Here's how the part is built. I have some questions about the finished solid (model axes, mm). A direction names the side the tool comes from. Coordinates: 2 decimals unless noted, no trailing zeros. Write each loop counter-clockwise with the first axis right and the second up, starting at its lowest first coordinate (ties: lowest second). Pieces come first, ordered by that corner, then holes.
Item 1: I want a section at C-C (y = -3). Please give me the cut outline in (x, z), and give its area (3 significant figures).
Item 2: I'm going to push flat-ended pins straight in: P1, Ø1.5, axis at x = 5, z = -1.5, coming from the -Y side; P2, Ø3, axis at y = -4, z = -2, coming from the -X side; P3, Ø1.5, axis at y = -18, z = 2.5, coming from the -X side; P4, Ø1, axis at y = 2, z = 1.5, coming from the -X side. Where does each tip first touch, or does it pass through?
Item 3: If we mould it in two halves opening along Y, with no side actions, what happens to faces 5 (the face through (-15, -7, 2)), 6 (the face through (-13.5, 5.07, 2.54)), 7 (the face through (10, -2, 1))? For each: pulls with the +Y half, pulls with the -Y half, needs draft (parallel to the pull), parting line crosses it, or undercut.
Item 4: I want a section at B-B (x = 18.5). Please give me the cut outline in (y, z), and give its area (3 significant figures).
Item 5: Please list where these lines run through material, in increasing order: line 1 (X direction, y = -13.5, z = 2.5); line 2 (X direction, y = -6.25, z = 1); line 3 (X direction, y = -7.75, z = 2).
Item 6: For faces 1 (the face through (8.4, -3.7, 3)), 2 (the face through (15.5, -3, -2)), 3 (the face through (-1, -14.5, 2)), 4 (the face through (8.84, -5.94, -1.97)), which set-ups out of +Z, -Z, +X, -X, +Y, -Y let a thin tool reach every point of the face, with its end or its side?
Item 7: I want a section at D-D (x = -7.5). Please give me the cut outline in (y, z), and give its area (3 significant figures).
from build123d import *

# Parameters (mm, degrees)
SKETCH1_W             = 23
SKETCH1_H             = 21
EXTRUDE1_DEPTH        = 5
SKETCH2_R             = 2.15
EXTRUDE2_DEPTH        = 4.3
SKETCH3_R             = 4.5
EXTRUDE3_DEPTH        = 4.5
SKETCH4_R             = 1.25
EXTRUDE4_DEPTH        = 8
SKETCH7_W             = 12
SKETCH7_H             = 26
EXTRUDE6_DEPTH        = 5
SKETCH9_R             = 1.5
EXTRUDE8_DEPTH        = 5
SKETCH8_R             = 2
EXTRUDE7_DEPTH        = 4
FILLET2_R             = 3
M3_TAPPED_HOLE1_D     = 2.5
M3_TAPPED_HOLE1_DEPTH = 8
M3_TAPPED_HOLE1_TIP   = 0.751075774
EXTRUDE9_DEPTH        = 4
FILLET1_R             = 5
EXTRUDE10_DEPTH       = 4
FILLET3_R             = 2


with BuildPart() as part:
    # Sketch1 → Extrude1 (new body)
    with BuildSketch(Plane.XY):
        with Locations((-3.5, -4)):
            Rectangle(SKETCH1_W, SKETCH1_H)
    extrude(amount=EXTRUDE1_DEPTH)

    # Sketch2 → Extrude2 (cut)
    with BuildSketch(Plane.XY.offset(5)):
        with Locations((-6, 0)):
            Circle(SKETCH2_R)
    extrude(amount=-EXTRUDE2_DEPTH, mode=Mode.SUBTRACT)

    # Sketch3 → Extrude3 (cut)
    with BuildSketch(Plane(origin=(0, 0, 0), x_dir=(-1, 0, 0), z_dir=(0, 0, -1))):
        with Locations((4.9, -6.5)):
            Circle(SKETCH3_R)
    extrude(amount=-EXTRUDE3_DEPTH, mode=Mode.SUBTRACT)

    # Sketch4 → Extrude4 (cut)
    with BuildSketch(Plane.XZ.offset(14.5)):
        with Locations(Location((-12, 2.5, 0), (0, 0, 270))):
            Circle(SKETCH4_R)
        with Locations(Location((1.4, 2.5, 0), (0, 0, 270))):
            Circle(SKETCH4_R)
    extrude(amount=-EXTRUDE4_DEPTH, mode=Mode.SUBTRACT)

    # Sketch7 → Extrude6 (add)
    with BuildSketch(Plane.XY.offset(5)):
        with Locations((14, -6.5)):
            Rectangle(SKETCH7_W, SKETCH7_H)
    extrude(amount=-EXTRUDE6_DEPTH)

    # Sketch9 → Extrude8 (cut)
    with BuildSketch(Plane.XY.offset(5)):
        with Locations((17.5, -5.5)):
            Circle(SKETCH9_R)
    extrude(amount=-EXTRUDE8_DEPTH, mode=Mode.SUBTRACT)

    # Sketch8 → Extrude7 (cut)
    with BuildSketch(Plane.XY.offset(5)):
        with Locations((10, -2.5)):
            Circle(SKETCH8_R)
    extrude(amount=-EXTRUDE7_DEPTH, mode=Mode.SUBTRACT)

    # Fillet2
    fillet2_edges = [part.edges().sort_by_distance(p)[0] for p in [
        (20, 6.5, 2.5),
        (20, -19.5, 2.5),
    ]]
    fillet(fillet2_edges, radius=FILLET2_R)

    # M3 Tapped Hole1
    with Locations(Plane(origin=(-12, -14.5, 2.5), x_dir=(0, 0, -1), z_dir=(0, -1, 0))):
        with Locations((0, 0), (0, 13.4)):
            Hole(M3_TAPPED_HOLE1_D / 2, depth=M3_TAPPED_HOLE1_DEPTH)
            with Locations((0, 0, -(M3_TAPPED_HOLE1_DEPTH + M3_TAPPED_HOLE1_TIP / 2))):  # 118° drill point
                Cone(0, M3_TAPPED_HOLE1_D / 2, M3_TAPPED_HOLE1_TIP, mode=Mode.SUBTRACT)

    # Sketch11 → Extrude9 (add)
    with BuildSketch(Plane(origin=(0, 0, 0), x_dir=(-1, 0, 0), z_dir=(0, 0, -1))):
        Polygon((-8, -19.5), (-20, -19.5), (-20, 1), (-18.1, 1), (-2, -11.07), (-2, -14.5), (-8, -14.5), align=None)
    extrude(amount=EXTRUDE9_DEPTH)

    # Fillet1
    fillet1_edges = [part.edges().sort_by_distance(p)[0] for p in [
        (-15, 6.5, 2.5),
        (20, -19.5, -2),
    ]]
    fillet(fillet1_edges, radius=FILLET1_R)

    # Sketch12 → Extrude10 (cut)
    with BuildSketch(Plane(origin=(0, 0, -4), x_dir=(-1, 0, 0), z_dir=(0, 0, -1))):
        Polygon((-19.5, 1), (-19.5, -7.5), (-15.5, -7.5), (-15.5, -0.949192547), (-18.1, 1), align=None)
    extrude(amount=-EXTRUDE10_DEPTH, mode=Mode.SUBTRACT)

    # Fillet3
    fillet3_edges = [part.edges().sort_by_distance(p)[0] for p in [
        (15.5, -7.5, -2),
        (19.5, -7.5, -2),
    ]]
    fillet(fillet3_edges, radius=FILLET3_R - 0.0001)  # a hair under: the kernel refuses the full size


solid = part.part
Answer:
1. outline: (-15, 0) - (-7.73, 0) - (-7.73, 4.5) - (-2.07, 4.5) - (-2.07, 0) - (12.76, 0) - (12.76, -4) - (15.5, -4) - (15.5, 0) - (19.5, 0) - (19.5, -4) - (20, -4) - (20, 5) - (11.94, 5) - (11.94, 1) - (8.06, 1) - (8.06, 5) - (-15, 5) - close
1. area: 147 mm2
2. P1: stops at y = -14.5
2. P2: stops at x = 9.43
2. P3: stops at x = 8
2. P4: stops at x = -15
3. face 5: needs draft
3. face 6: pulls with the +Y half
3. face 7: undercut
4. outline: (-18.07, -4) - (-7.23, -4) - (-7.23, 0) - (-6.62, 0) - (-6.62, 5) - (-18.07, 5) - close; (-4.38, 0) - (6.1, 0) - (6.1, 5) - (-4.38, 5) - close
4. area: 153 mm2
5. line 1: x = -15 to -13.25, -10.75 to 0.15, 2.65 to 20
5. line 2: x = -15 to -9.39, -0.41 to 16.2, 18.8 to 20
5. line 3: x = -15 to -13.15, -10.85 to -9.22, -0.58 to 0.25, 2.55 to 20
6. face 1: +Z
6. face 2: -Z, +Y
6. face 3: +Z, -Z, -X, -Y
6. face 4: -Z, -X, +Y
7. outline: (-14.5, 0) - (-10.17, 0) - (-10.17, 4.5) - (-2.83, 4.5) - (-2.83, 0) - (6.5, 0) - (6.5, 5) - (1.54, 5) - (1.54, 0.7) - (-1.54, 0.7) - (-1.54, 5) - (-14.5, 5) - close
7. area: 58.7 mm2
